from build123d import *

# Parameters (mm, degrees)
F0_R     = 14
F1_DEPTH = 25


with BuildPart() as f1:
    # F0 (on Top) → F1 (new body)
    with BuildSketch(Plane.XY):
        with BuildLine():
            ThreePointArc((21.863849, -5.004198), (16.734289, 7.468286), (21.708714, 20.003449))
            ThreePointArc((21.708714, 20.003449), (-9.013445, 69.323231), (-5.922247, 11.299646))
            Line((-5.922247, 11.299646), (1.68415, -9.262297))
            Line((1.68415, -9.262297), (25, -72.290713))
            ThreePointArc((25, -72.290713), (0, -97.290713), (-25, -72.290713))
            Line((-25, -72.290713), (-38.807588, -56.926059))
            ThreePointArc((-38.807588, -56.926059), (-41.028289, -54.254293), (-43.036256, -51.419171))
            ThreePointArc((-43.036256, -51.419171), (-54.45074, -49.322706), (-55.948149, -60.831111))
            ThreePointArc((-55.948149, -60.831111), (-19.496759, -129.623891), (54.195657, -104.512574))
            ThreePointArc((54.195657, -104.512574), (60.796806, -88.998974), (63.050913, -72.290713))
            ThreePointArc((63.050913, -72.290713), (56.997606, -45.333515), (40, -23.552457))
            Line((40, -23.552457), (21.863849, -5.004198))
        make_face()
        with Locations((0, 40.709287)):
            Circle(F0_R, mode=Mode.SUBTRACT)
    extrude(amount=F1_DEPTH)


solid = f1.part
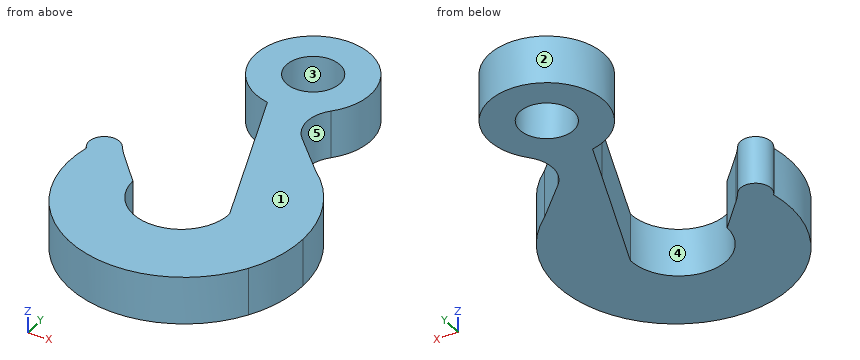
The listing builds one solid part. Answer for the finished solid, in the listing's coordinates (mm). Face numbers are marked on the shaded views. A direction names the side the tool comes from. Round coordinates to 2 decimals unless told otherwise and drop trailing zeros. Order: outer loops, then holes, each group sorted by start corner. A loop starts at its lowest first (then second) coordinate and runs counter-clockwise, first axis right, second up. Notation, with made-up numbers: M -17,42.25 L 16,42.25 A13 ccw 16,55.25 Z; hole C 0.5,10 d8. An arc over 180 degrees is marked long. Answer in a Markdown table with one row per item. Add a question column.
1) Flat-ended cylindrical pins translate along their axes: pin 1 Ø5 at (y, z) = (-37, 17.5) entering from +X; pin 2 Ø5 at (y, z) = (-27.5, 17) entering from +X; pin 3 Ø4 at (y, z) = (-10.5, 18) entering from -X. Find the tip coordinate at first contact, or state that the pin passes through.
2) The part is cut by section A-A on x = -2.5. Determine the outline of the cut face in (y, z), plus the area to 3 significant figures.
3) Determine the mould class of the marked faces 1, 2 and 3 for opening direction X: pulls with the +X half, pulls with the -X half, needs draft (parallel to the pull), parting line crosses it, or undercut.
4) Consider line 1 along X through (y, z) = (42.5, 20.75) (1 decimal); line 2 along X through (y, z) = (-50, 9); line 3 along X through (y, z) = (2, 6.5). Determine where each line is inside the solid, lowest interval first. Write a range as from..to.
5) The part is cut by section C-C on y = -37. Determine the outline of the cut face in (x, z), plus the area to 3 significant figures.
6) Which of the six approach directions +Z, -Z, +X, -X, +Y, -Y give full straight-line access (tool end or side, diameter ignored) to the marked faces 4 and 5?
7) The part is cut by section B-B on z = 3. Determine the outline of the cut face in (x, y), plus the area to 3 significant figures.
8) The part is cut by section D-D on x = 33. Determine the outline of the cut face in (y, z).
Findings below:
| question | item | result |
|---|---|---|
| 1 | pin 1 | stops at x = 53.85 |
| 1 | pin 2 | stops at x = 46.76 |
| 1 | pin 3 | stops at x = 1.4 |
| 2 | outline | M -133.63,0 L -97.17,0 L -97.17,25 L -133.63,25 Z; M 2.05,0 L 26.93,0 L 26.93,25 L 2.05,25 Z; M 54.48,0 L 70.6,0 L 70.6,25 L 54.48,25 Z |
| 2 | area | 1,940 mm² |
| 3 | face 1 | needs draft |
| 3 | face 2 | parting line crosses it |
| 3 | face 3 | undercut |
| 4 | line 1 | x = -29.9..-13.9, 13.9..29.9 |
| 4 | line 2 | x = -55.26..-44.22, 16.75..58.98 |
| 4 | line 3 | x = -2.48..17.62 |
| 5 | outline | M 11.95,0 L 52.25,0 L 52.25,25 L 11.95,25 Z |
| 5 | area | 1,010 mm² |
| 6 | face 4 | +Z, -Z |
| 6 | face 5 | +Z, -Z, +X |
| 7 | outline | M -55.95,-60.83 A60 ccw 54.2,-104.51 A63.05 ccw 63.05,-72.29 A63.05 ccw 40,-23.55 L 21.86,-5 A18 cw 21.71,20 A30 ccw long -5.92,11.3 L 25,-72.29 A25 cw -25,-72.29 L -38.81,-56.93 A45 cw -43.04,-51.42 A8 ccw long Z; hole C 0,40.71 d28 |
| 7 | area | 10,400 mm² |
| 8 | outline | M -125.59,0 L -16.39,0 L -16.39,25 L -125.59,25 Z |
